```python
from build123d import *

# Parameters (mm, degrees)
SKETCH1_W           = 32.6
SKETCH1_H           = 32.6
BOSS_EXTRUDE1_DEPTH = 1.2
SKETCH3_R           = 1.075
CUT_EXTRUDE1_DEPTH  = 24.082894099
SKETCH4_W           = 17
SKETCH4_H           = 17
BOSS_EXTRUDE2_DEPTH = 7.9
BOSS_EXTRUDE3_DEPTH = 7.9
SKETCH6_R           = 7.8
BOSS_EXTRUDE4_DEPTH = 5.9
SKETCH7_R           = 5.95
BOSS_EXTRUDE5_DEPTH = 6.6
SKETCH8_R           = 7
BOSS_EXTRUDE6_DEPTH = 3.3


with BuildPart() as part:
    # Sketch1 → Boss-Extrude1 (new body)
    with BuildSketch(Plane.XY):
        Rectangle(SKETCH1_W, SKETCH1_H)
    extrude(amount=BOSS_EXTRUDE1_DEPTH)

    # Sketch3 → Cut-Extrude1 (cut, through all)
    with BuildSketch(Plane.XY.offset(1.2)):
        with Locations((-14.25, 14.25)):
            Circle(SKETCH3_R)
        with Locations((14.25, 14.25)):
            Circle(SKETCH3_R)
        with Locations((14.25, -14.25)):
            Circle(SKETCH3_R)
        with Locations((-14.25, -14.25)):
            Circle(SKETCH3_R)
    extrude(amount=-CUT_EXTRUDE1_DEPTH, mode=Mode.SUBTRACT)

    # Sketch4 → Boss-Extrude2 (add)
    with BuildSketch(Plane.XY.offset(1.2)):
        Rectangle(SKETCH4_W, SKETCH4_H)
    extrude(amount=BOSS_EXTRUDE2_DEPTH)

    # Sketch5 → Boss-Extrude3 (add)
    with BuildSketch(Plane.XY.offset(1.2)):
        with BuildLine():
            Line((-10, 2.4), (10, 2.4))
            ThreePointArc((10, 2.4), (12.4, 0), (10, -2.4))
            Line((10, -2.4), (-10, -2.4))
            ThreePointArc((-10, -2.4), (-12.4, 0), (-10, 2.4))
        make_face()
    extrude(amount=BOSS_EXTRUDE3_DEPTH)

    # Sketch6 → Boss-Extrude4 (add)
    with BuildSketch(Plane.XY.offset(9.1)):
        Circle(SKETCH6_R)
    extrude(amount=BOSS_EXTRUDE4_DEPTH)

    # Sketch7 → Boss-Extrude5 (add)
    with BuildSketch(Plane.XY.offset(15)):
        Circle(SKETCH7_R)
    extrude(amount=BOSS_EXTRUDE5_DEPTH)

    # Sketch8 → Boss-Extrude6 (add)
    with BuildSketch(Plane.XY.offset(21.6)):
        Circle(SKETCH8_R)
    extrude(amount=BOSS_EXTRUDE6_DEPTH)


solid = part.part
```
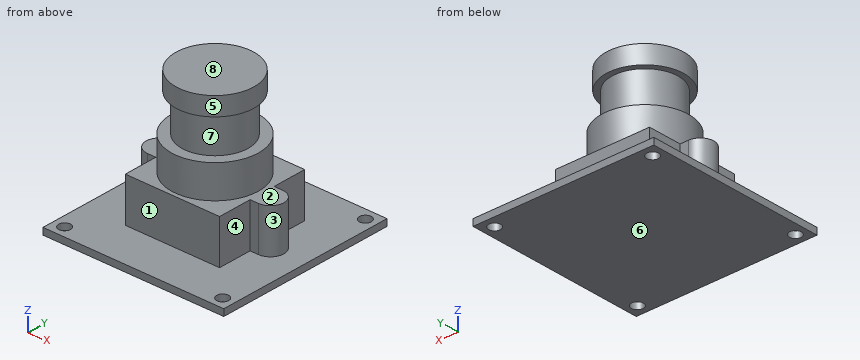
Model file for the job. Use its own axes, mm. Face numbers are marked on the shaded views. A direction names the side the tool comes from. Give positions to 0.01 mm unless a question says otherwise; leave off trailing zeros. Order: outer loops, then holes, each group sorted by start corner. A loop starts at its lowest first (then second) coordinate and runs counter-clockwise, first axis right, second up.
1) Mould opens along Z. For the marked faces 5, 6, 7 and 8 say: +Z half, -Z half, draft (parallel to the pull), parting line (faces both ways), or undercut.
2) Saw through at D-D, the plane x = 0. Write the cut outline in (y, z).
3) Pin check, flat tips, straight feed: pin 1 (1.8 mm diameter, centred on y = -5, z = 6.5, fed in from -X); pin 2 (1.6 mm diameter, centred on x = 9.5, z = 7, fed in from +Y); pin 3 (8.5 mm diameter, centred on x = 0.5, z = 6.5, fed in from +Y). Stop position of each tip, or through.
4) 3-axis set-ups, long thin cutter, end or side, ignore diameter. For the marked faces 1, 2, 3 and 4: which of +Z, -Z, +X, -X, +Y, -Y reach the whole face in a straight line?
5) Saw through at A-A, the plane x = 14.25. Write the cut outline in (y, z) (3 decimals), then the cut area to 3 significant figures.
6) Saw through at C-C, the plane z = 6.5. Write the cut outline in (x, y), then the cut area to 3 significant figures.
7) Wall check: probe 1 along Y at (x, z) = (-14.25, 0.7) (3 decimals); probe 2 along Z at (x, y) = (3.5, -5.5); probe 3 along Z at (x, y) = (-12.5, -12). Give the ranges that are in metal, low to high.
Computed:
1. face 5: draft
1. face 6: -Z half
1. face 7: undercut
1. face 8: +Z half
2. outline: (-16.3, 0) - (16.3, 0) - (16.3, 1.2) - (8.5, 1.2) - (8.5, 9.1) - (7.8, 9.1) - (7.8, 15) - (5.95, 15) - (5.95, 21.6) - (7, 21.6) - (7, 24.9) - (-7, 24.9) - (-7, 21.6) - (-5.95, 21.6) - (-5.95, 15) - (-7.8, 15) - (-7.8, 9.1) - (-8.5, 9.1) - (-8.5, 1.2) - (-16.3, 1.2) - close
3. pin 1: stops at x = -8.5
3. pin 2: stops at y = 2.4
3. pin 3: stops at y = 8.5
4. face 1: +Z, +X, -X, -Y
4. face 2: +Z
4. face 3: +Z, +X
4. face 4: +Z, +X, -Y
5. outline: (-16.3, 0) - (-15.325, 0) - (-15.325, 1.2) - (-16.3, 1.2) - close; (-13.175, 0) - (13.175, 0) - (13.175, 1.2) - (-13.175, 1.2) - close; (15.325, 0) - (16.3, 0) - (16.3, 1.2) - (15.325, 1.2) - close
5. area: 34.0 mm2
6. outline: (-10, -2.4) - (-8.5, -2.4) - (-8.5, -8.5) - (8.5, -8.5) - (8.5, -2.4) - (10, -2.4) arc R2.4 ccw to (10, 2.4) - (8.5, 2.4) - (8.5, 8.5) - (-8.5, 8.5) - (-8.5, 2.4) - (-10, 2.4) arc R2.4 ccw to start
6. area: 321 mm2
7. probe 1: y = -16.3 to -15.325, -13.175 to 13.175, 15.325 to 16.3
7. probe 2: z = 0 to 15, 21.6 to 24.9
7. probe 3: z = 0 to 1.2
